```python
from build123d import *

# Parameters (mm, degrees)
SKETCH1_W           = 61
SKETCH1_H           = 100
BOSS_EXTRUDE1_DEPTH = 80
SKETCH2_OUTSIDE_W   = 110.37
SKETCH2_OUTSIDE_H   = 130.37
CUT_EXTRUDE1_DEPTH  = 113.343224095
SKETCH3_W           = 51
SKETCH3_H           = 90
CUT_EXTRUDE2_DEPTH  = 100.147617218
SKETCH4_W           = 51
SKETCH4_H           = 10
CUT_EXTRUDE3_DEPTH  = 125.21855739
FILLET3_R           = 5
FILLET4_R           = 5
SKETCH5_R           = 3.5
CUT_EXTRUDE4_DEPTH  = 117.147842498


with BuildPart() as part:
    # Sketch1 → Boss-Extrude1 (new body)
    with BuildSketch(Plane.XY):
        Rectangle(SKETCH1_W, SKETCH1_H)
    extrude(amount=-BOSS_EXTRUDE1_DEPTH)

    # Sketch2 outside → Cut-Extrude1 (cut, through all)
    with BuildSketch(Plane.ZY.offset(30.5)):
        with Locations((-40, 0)):
            Rectangle(SKETCH2_OUTSIDE_W, SKETCH2_OUTSIDE_H)
        Polygon((-80, -25), (-50, -25), (0, 50), (0, -50), (-80, -50), align=None, mode=Mode.SUBTRACT)
    extrude(amount=-CUT_EXTRUDE1_DEPTH, mode=Mode.SUBTRACT)

    # Sketch3 → Cut-Extrude2 (cut, through all)
    with BuildSketch(Plane.XY):
        with Locations((0, 5)):
            Rectangle(SKETCH3_W, SKETCH3_H)
    extrude(amount=-CUT_EXTRUDE2_DEPTH, mode=Mode.SUBTRACT)

    # Sketch4 → Cut-Extrude3 (cut, through all)
    with BuildSketch(Plane(origin=(0, -40, 0), x_dir=(1, 0, 0), z_dir=(0, 1, 0))):
        with Locations((0, 5)):
            Rectangle(SKETCH4_W, SKETCH4_H)
    extrude(amount=-CUT_EXTRUDE3_DEPTH, mode=Mode.SUBTRACT)

    # Sketch9_8 → Cut-Revolve4 (revolve, cut)
    with BuildSketch(Plane.XY.offset(-10)):
        Polygon((-23.4, 14), (-30.5, 6.9), (-30.5, 14), align=None)
    cut_revolve4 = revolve(axis=Axis((-30.5, 14, -10), (1, 0, 0)), mode=Mode.SUBTRACT)

    # Sketch9_9 → Cut-Revolve5 (revolve, cut)
    with BuildSketch(Plane.XY.offset(-10), mode=Mode.PRIVATE) as cut_revolve5_sk:
        Polygon((-23.4, -30), (-30.5, -37.1), (-30.5, -30), align=None)
    cut_revolve5 = revolve(cut_revolve5_sk.sketch.rotate(Axis((-30.5, -30, -10), (1, 0, 0)), 270), axis=Axis((-30.5, -30, -10), (1, 0, 0)), mode=Mode.SUBTRACT)

    # Mirror1: Cut-Revolve4, Cut-Revolve5 across plane
    add(cut_revolve4.mirror(Plane(origin=(0, 0, 0), x_dir=(0, 0, 1), z_dir=(1, 0, 0))), mode=Mode.SUBTRACT)
    add(cut_revolve5.mirror(Plane(origin=(0, 0, 0), x_dir=(0, 0, 1), z_dir=(1, 0, 0))), mode=Mode.SUBTRACT)

    # Fillet3
    fillet3_edges = [part.edges().sort_by_distance(p)[0] for p in [
        (-28, 50, 0),
        (28, 50, 0),
    ]]
    fillet(fillet3_edges, radius=FILLET3_R)

    # Fillet4
    fillet4_edges = [part.edges().sort_by_distance(p)[0] for p in [
        (28, -25, -80),
        (28, -25, -50),
        (-28, -25, -50),
        (-28, -25, -80),
    ]]
    fillet(fillet4_edges, radius=FILLET4_R)

    # Sketch5 → Cut-Extrude4 (cut, through all)
    with BuildSketch(Plane(origin=(0, -40, 0), x_dir=(1, 0, 0), z_dir=(0, 1, 0))):
        with Locations(Location((0, 55, 0), (0, 0, 180))):
            Circle(SKETCH5_R)
    extrude(amount=-CUT_EXTRUDE4_DEPTH, mode=Mode.SUBTRACT)


solid = part.part
```
Verification items for the finished model (mm, model axes). A direction names the side the tool comes from. Round coordinates to 2 decimals unless told otherwise and drop trailing zeros. Write each loop counter-clockwise with the first axis right and the second up, starting at its lowest first coordinate (ties: lowest second). Pieces come first, ordered by that corner, then holes.
1. Section check A-A on y = 14. Enter the section's corners in (x, z).
2. Section check D-D on z = -60. Enter the section's corners in (x, y).
3. Gauge pin test, flat ends, axial feed: P1, Ø2.5, axis at x = 29, z = -61, coming from the +Y side; P2, Ø3, axis at x = 1, y = -42.5, coming from the +Z side; P3, Ø11, axis at x = 0, z = -55, coming from the +Y side. Record the tip position at first contact, or that the pin passes through.
4. Section check B-B on x = 0. Enter the section's corners in (y, z), plus the area to 3 significant figures.
5. Scan lines: L1, parallel to X at y = -37, z = -70; L2, parallel to Z at x = 0, y = -42; L3, parallel to Y at x = -17, z = -51.5. Record each from-to range of solid material in increasing order.
6. Access from +Z, -Z, +X, -X, +Y, -Y to the whole of each face (thin tool, end or side, straight path). Record for faces 1 (the flat face through (-28, -25, -64)), 2 (the flat face through (-28, -8, 0)), 3 (the flat face through (0, -45, -10)).
7. Section check C-C on y = 31.5. Enter the section's corners in (x, z).
8. Draft check along Z on faces 4 (the flat face through (28, -25, -64)), 5 (the conical face through (-25.81, 11.7, -10.72)), 6 (the cylindrical face through (-28, -27, -79)). Enter one of: +Z half, -Z half, draft (parallel to the pull), parting line (faces both ways), or undercut.
Answer:
1. outline: (-30.5, -24) - (-25.5, -24) - (-25.5, -12.1) - (-30.5, -17.1) - close; (-30.5, -2.9) - (-25.5, -7.9) - (-25.5, 0) - (-30.5, 0) - close; (25.5, -24) - (30.5, -24) - (30.5, -17.1) - (25.5, -12.1) - close; (25.5, -7.9) - (30.5, -2.9) - (30.5, 0) - (25.5, 0) - close
2. outline: (-30.5, -50) - (30.5, -50) - (30.5, -25) - (25.5, -25) - (25.5, -40) - (-25.5, -40) - (-25.5, -25) - (-30.5, -25) - close
3. P1: stops at y = -25
3. P2: stops at z = -10
3. P3: stops at y = -40
4. outline: (-50, -80) - (-40, -80) - (-40, -58.5) - (-50, -58.5) - close; (-50, -51.5) - (-40, -51.5) - (-40, -10) - (-50, -10) - close
4. area: 630 mm2
5. L1: x = -30.5 to -25.5, 25.5 to 30.5
5. L2: z = -80 to -58.5, -51.5 to -10
5. L3: y = -50 to -40
6. face 1: -Z, +X, -X, +Y
6. face 2: +Z, +X, -X, +Y, -Y
6. face 3: +Z, +Y, -Y
7. outline: (-30.5, -12.33) - (-25.5, -12.33) - (-25.5, 0) - (-30.5, 0) - close; (25.5, -12.33) - (30.5, -12.33) - (30.5, 0) - (25.5, 0) - close
8. face 4: draft
8. face 5: undercut
8. face 6: -Z half
